Autodesk Fusion 360 part; units mm, degrees
sketch "Sketch1" plane through (0, 0, 0) normal (0, 0, 1) x (1, 0, 0)
  line L0 (-1, 0) -> (-71, 0)
  line L1 (-72, -1) -> (-72, -24)
  line L2 (-71, -25) -> (-1, -25)
  line L3 (0, -24) -> (0, -1)
  arc A0 (-1, -25) -> (0, -24) centre (-1, -24) ccw
  arc A1 (-72, -24) -> (-71, -25) centre (-71, -24) ccw
  arc A2 (-71, 0) -> (-72, -1) centre (-71, -1) ccw
  arc A3 (0, -1) -> (-1, 0) centre (-1, -1) ccw
  line L4 (2, -24) -> (2, -1)
  arc A4 (2, -1) -> (-1, 2) centre (-1, -1) ccw
  line L5 (-1, 2) -> (-71, 2)
  arc A5 (-71, 2) -> (-74, -1) centre (-71, -1) ccw
  line L6 (-74, -1) -> (-74, -24)
  arc A6 (-74, -24) -> (-71, -27) centre (-71, -24) ccw
  line L7 (-71, -27) -> (-1, -27)
  arc A7 (-1, -27) -> (2, -24) centre (-1, -24) ccw
  point P0 (-72, 0)
  point P1 (0, -25)
  dimension "d1" = 72
  dimension "d2" = 25
  dimension "d3" = 1
  dimension "d4" = 2
extrude "Extrude1" add sketch "Sketch1" along normal blind 3
sketch "Sketch2" plane through (0, 0, 3) normal (0, 0, 1) x (-1, 0, 0)
  arc A0 (0, 1) -> (1, 0) centre (1, 1) ccw
  line L0 (0, 1) -> (0, 24)
  arc A1 (1, 25) -> (0, 24) centre (1, 24) ccw
  line L1 (1, 25) -> (71, 25)
  arc A2 (72, 24) -> (71, 25) centre (71, 24) ccw
  line L2 (72, 24) -> (72, 1)
  arc A3 (71, 0) -> (72, 1) centre (71, 1) ccw
  line L3 (71, 0) -> (1, 0)
  arc A4 (1, 27) -> (-2, 24) centre (1, 24) ccw
  line L4 (-2, 24) -> (-2, 1)
  arc A5 (-2, 1) -> (1, -2) centre (1, 1) ccw
  line L5 (1, -2) -> (71, -2)
  arc A6 (71, -2) -> (74, 1) centre (71, 1) ccw
  line L6 (74, 1) -> (74, 24)
  arc A7 (74, 24) -> (71, 27) centre (71, 24) ccw
  line L7 (71, 27) -> (1, 27)
  line L8 (71, 27) -> (1, 27)
  line L9 (6.5, 19.5) -> (65.5, 19.5)
  line L10 (5.5, 6.5) -> (5.5, 18.5)
  line L11 (65.5, 5.5) -> (6.5, 5.5)
  line L12 (66.5, 18.5) -> (66.5, 6.5)
  arc A8 (6.5, 19.5) -> (5.5, 18.5) centre (6.5, 18.5) ccw
  arc A9 (66.5, 18.5) -> (65.5, 19.5) centre (65.5, 18.5) ccw
  arc A10 (65.5, 5.5) -> (66.5, 6.5) centre (65.5, 6.5) ccw
  arc A11 (5.5, 6.5) -> (6.5, 5.5) centre (6.5, 6.5) ccw
  dimension "d8" = 1
extrude "Extrude2" add sketch "Sketch2" along normal blind 1 contours A0 L0 A1 L1 A2 L2 A3 L3 | A4 L4 A5 L5 A6 L6 A7 L7 L8
fillet "Fillet1" radius 0.5 8 edges at (-66.5, -12.5, 4) (-66.2071, -5.7929, 4) (-36, -5.5, 4) (-5.7929, -5.7929, 4) (-5.5, -12.5, 4) (-5.7929, -19.2071, 4) (-36, -19.5, 4) (-66.2071, -19.2071, 4)
fillet "Fillet2" radius 0.5 8 edges at (-73.1213, 1.1213, 4) (-74, -12.5, 4) (-73.1213, -26.1213, 4) (-36, -27, 4) (1.1213, -26.1213, 4) (2, -12.5, 4) (1.1213, 1.1213, 4) (-36, 2, 4)
sketch "Sketch3" plane through (0, 0, 4) normal (0, 0, 1) x (-1, 0, 0)
  line L0 (67, 18.5) -> (67, 6.5)
  arc A0 (65.5, 5) -> (67, 6.5) centre (65.5, 6.5) ccw
  line L1 (65.5, 5) -> (6.5, 5)
  arc A1 (5, 6.5) -> (6.5, 5) centre (6.5, 6.5) ccw
  line L2 (5, 6.5) -> (5, 18.5)
  arc A2 (6.5, 20) -> (5, 18.5) centre (6.5, 18.5) ccw
  line L3 (6.5, 20) -> (65.5, 20)
  arc A3 (67, 18.5) -> (65.5, 20) centre (65.5, 18.5) ccw
  arc A4 (71, -1.5) -> (73.5, 1) centre (71, 1) ccw
  line L4 (73.5, 1) -> (73.5, 24)
  arc A5 (73.5, 24) -> (71, 26.5) centre (71, 24) ccw
  line L5 (71, 26.5) -> (1, 26.5)
  arc A6 (1, 26.5) -> (-1.5, 24) centre (1, 24) ccw
  line L6 (-1.5, 24) -> (-1.5, 1)
  arc A7 (-1.5, 1) -> (1, -1.5) centre (1, 1) ccw
  line L7 (1, -1.5) -> (71, -1.5)
  line L8 (0.5, 24) -> (0.5, 1)
  arc A8 (0.5, 1) -> (1, 0.5) centre (1, 1) ccw
  line L9 (1, 0.5) -> (71, 0.5)
  arc A9 (71, 0.5) -> (71.5, 1) centre (71, 1) ccw
  line L10 (71.5, 1) -> (71.5, 24)
  arc A10 (71.5, 24) -> (71, 24.5) centre (71, 24) ccw
  line L11 (71, 24.5) -> (1, 24.5)
  arc A11 (1, 24.5) -> (0.5, 24) centre (1, 24) ccw
  arc A12 (3, 6.5) -> (6.5, 3) centre (6.5, 6.5) ccw
  line L12 (65.5, 3) -> (6.5, 3)
  arc A13 (65.5, 3) -> (69, 6.5) centre (65.5, 6.5) ccw
  line L13 (69, 18.5) -> (69, 6.5)
  arc A14 (69, 18.5) -> (65.5, 22) centre (65.5, 18.5) ccw
  line L14 (6.5, 22) -> (65.5, 22)
  arc A15 (6.5, 22) -> (3, 18.5) centre (6.5, 18.5) ccw
  line L15 (3, 6.5) -> (3, 18.5)
  dimension "d15" = -2
  dimension "d16" = -2
extrude "Extrude3" add sketch "Sketch3" along normal blind 1 contours L8 A8 L9 A9 L10 A10 L11 A11
fillet "Fillet3" radius 0.75 16 edges at (-67.9749, -20.9749, 5) (-69, -12.5, 5) (-67.9749, -4.0251, 5) (-36, -3, 5) (-4.0251, -4.0251, 5) (-3, -12.5, 5) (-4.0251, -20.9749, 5) (-36, -22, 5) (-36, -0.5, 5) (-71.3536, -0.6464, 5) (-71.5, -12.5, 5) (-71.3536, -24.3536, 5) (-36, -24.5, 5) (-0.6464, -24.3536, 5) (-0.5, -12.5, 5) (-0.6464, -0.6464, 5)
Can you work these out from the model? Positions are in its coordinate system, mm. A direction names the side the tool comes from. Give positions to 0.01 mm unless a question says otherwise; leave off trailing zeros. Order: outer loops, then holes, each group sorted by start corner. A loop starts at its lowest first (then second) coordinate and runs counter-clockwise, first axis right, second up. Notation, with made-up numbers: (-31, 62) - (17, 62) arc R25 ccw to (17, 92) - close; hole circle Ø5 at (43.5, 71). An arc over 180 degrees is marked (long way). Write each question's results on one line, items separated by ' | '.
1) If we mould it in two halves opening along Y, with no side actions, what happens to faces 4 (the face through (-73.1, -26.14, 1.73)), 5 (the face through (-36.2, -25.3, 0)), 6 (the face through (-35.8, -20.3, 4))? For each: pulls with the +Y half, pulls with the -Y half, needs draft (parallel to the pull), parting line crosses it, or undercut.
Final values:
face 4: pulls with the -Y half | face 5: needs draft | face 6: undercut
2) Suppose I cut it at B-B, the plane z = 2. Write out the boundary of the cut face in (x, y), then the cut area to 3 significant figures.
Final values:
outline: (-74, -24) arc R3 ccw to (-71, -27) - (-1, -27) arc R3 ccw to (2, -24) - (2, -1) arc R3 ccw to (-1, 2) - (-71, 2) arc R3 ccw to (-74, -1) - close; hole (-72, -24) arc R1 ccw to (-71, -25) - (-1, -25) arc R1 ccw to (0, -24) - (0, -1) arc R1 ccw to (-1, 0) - (-71, 0) arc R1 ccw to (-72, -1) - close | area: 397 mm^2
3) I'm going to push flat-ended pins straight in: pin 1 Ø12 at (x, y) = (-28, -6.5) entering from -Z; pin 2 Ø4 at (x, y) = (-60.5, -3.5) entering from +Z; pin 3 Ø9.5 at (x, y) = (-25, -16.5) entering from +Z. Where does each tip first touch, or does it pass through?
Final values:
pin 1: stops at z = 3 | pin 2: stops at z = 5 | pin 3: stops at z = 4
4) Suppose I cut it at C-C, the plane y = -17.5. Write out the boundary of the cut face in (x, z).
Final values:
outline: (-74, 0) - (-72, 0) - (-72, 3) - (-66.5, 3) - (-66.5, 3.5) arc R0.5 ccw to (-67, 4) - (-69, 4) - (-69, 4.25) arc R0.75 ccw to (-69.75, 5) - (-70.75, 5) arc R0.75 ccw to (-71.5, 4.25) - (-71.5, 4) - (-73.5, 4) arc R0.5 ccw to (-74, 3.5) - close; (-5.5, 3) - (0, 3) - (0, 0) - (2, 0) - (2, 3.5) arc R0.5 ccw to (1.5, 4) - (-0.5, 4) - (-0.5, 4.25) arc R0.75 ccw to (-1.25, 5) - (-2.25, 5) arc R0.75 ccw to (-3, 4.25) - (-3, 4) - (-5, 4) arc R0.5 ccw to (-5.5, 3.5) - close
5) Suppose I cut it at A-A, the plane x = -32. Write out the boundary of the cut face in (y, z), then the cut area to 3 significant figures.
Final values:
outline: (-27, 0) - (-25, 0) - (-25, 3) - (-19.5, 3) - (-19.5, 3.5) arc R0.5 ccw to (-20, 4) - (-22, 4) - (-22, 4.25) arc R0.75 ccw to (-22.75, 5) - (-23.75, 5) arc R0.75 ccw to (-24.5, 4.25) - (-24.5, 4) - (-26.5, 4) arc R0.5 ccw to (-27, 3.5) - close; (-5.5, 3) - (0, 3) - (0, 0) - (2, 0) - (2, 3.5) arc R0.5 ccw to (1.5, 4) - (-0.5, 4) - (-0.5, 4.25) arc R0.75 ccw to (-1.25, 5) - (-2.25, 5) arc R0.75 ccw to (-3, 4.25) - (-3, 4) - (-5, 4) arc R0.5 ccw to (-5.5, 3.5) - close | area: 31.3 mm^2
6) On a 3-axis mill with a long thin cutter (end or side, diameter ignored), from which of +Z, -Z, +X, -X, +Y, -Y can I reach the whole of each face in a straight line? I mean faces 1 (the face through (-33, 0, 4)), 2 (the face through (-73.14, 1.1, 1.73)), 3 (the face through (-72, -12, 1)). Say none if no direction works.
Final values:
face 1: +Z | face 2: +Z, -Z, -X, +Y | face 3: -Z
7) Please list where these lines run through material, in increasing order: line 1 along Y through (x, z) = (-58.5, 2.05); line 2 along X through (y, z) = (-10.5, 2.7); line 3 along Y through (x, z) = (-60, 3.4). Write a range as [from, to].
Final values:
line 1: y = [-27, -25], [0, 2] | line 2: x = [-74, -72], [0, 2] | line 3: y = [-27, -19.5], [-5.5, 2]
